Source: CAD feature listing. Evaluate the final solid. Frame: model axes, mm. A direction names the side the tool comes from. Round coordinates to 2 decimals unless told otherwise and drop trailing zeros. Order: outer loops, then holes, each group sorted by start corner. A loop starts at its lowest first (then second) coordinate and runs counter-clockwise, first axis right, second up. Notation, with made-up numbers: (27.5, 21) -> (35.5, 21) arc R28 cw to (35.5, 54) -> close; hole circle Ø4 at (-26.75, 1). An arc over 180 degrees is marked (long way). Write item = value, one per line. Start each with the question number.
(1) Cut plane C-C on y = 9.75. Return the cut outline in (x, z) (1 decimal).
(2) Draft query along X for faces 1 (the face through (31.8, -1.29, -38.16)), 2 (the face through (40, -1.787, -21)), 3 (the face through (28.797, 4.855, -34.608)). Return one class per face: released by +X, released by -X, zero draft, split by the parting line, or undercut.
(3) Cut plane A-A on y = 1.5. Give the number of separate pieces and of enclosed holes in the cut face, then the cut area to 3 significant figures.
(4) Cut plane B-B on x = 16. Return the cut outline in (y, z), then the cut area to 3 significant figures.
(5) Ray query, line 1 (X direction, y = 7, z = -19); line 2 (X direction, y = 1.5, z = -27.5); line 3 (Z direction, x = 21, y = 13.25). Return the intervals inside material, ascending.
(6) Contact query for flat-ended pins moving along their axis: pin 1 Ø6 at (y, z) = (10.5, -29.5) entering from -X; pin 2 Ø5.5 at (y, z) = (5.5, -22) entering from -X; pin 3 Ø1.4 at (x, z) = (4.5, -21.5) entering from +Y; pin 4 Ø4 at (x, z) = (8.5, -29) entering from +Y. Output: stop coordinate, or through.
(7) Reachability of faces 4 (the face through (30, 9.037, -6)), 5 (the face through (31.794, -1.294, -3.731)), 6 (the face through (14.534, 3.992, -13.953)) from +Z, -Z, +X, -X, +Y, -Y: full face, straight path, thin tool, end or side. Return the list, or none.
from build123d import *

# Parameters (mm, degrees)
BOSS_EXTRUDE1_DEPTH         = 0.7874
BOSS_EXTRUDE1_DEPTH_BACK    = 0.7874
SKETCH1_R                   = 20.955
SKETCH2_R                   = 1.8034
BOSS_EXTRUDE2_DEPTH         = 2.54
SKETCH3_R                   = 0.44958
BOSS_EXTRUDE3_DEPTH         = 12.7
CIRPATTERN1_COUNT           = 3
SKETCH4_R                   = 9.5
BOSS_EXTRUDE4_DEPTH         = 6.5
SKETCH5_W                   = 2.8
SKETCH5_H                   = 5
BOSS_EXTRUDE5_DEPTH         = 8.25
SKETCH6_R                   = 2
BOSS_EXTRUDE6_DEPTH         = 5.5
REVOLVE1_ANGLE              = 90
CIRPATTERN2_COUNT           = 6
SKETCH8_W                   = 1
SKETCH8_H                   = 3
BOSS_EXTRUDE7_DEPTH         = 1
SKETCH9_W                   = 2
SKETCH9_H                   = 2
BOSS_EXTRUDE8_DEPTH         = 1
FILLET1_R                   = 0.75
CIRPATTERN3_COUNT           = 6
FILLET1_OF_CIRPATTERN3_R    = 0.75
SKETCH11_W                  = 0.762
SKETCH11_H                  = 0.01
BOSS_EXTRUDE10_DEPTH        = 1.5748
CIRPATTERN4_COUNT           = 2
CIRPATTERN4_ANGLE           = 3.4725
CIRPATTERN5_COUNT           = 2
CIRPATTERN5_ANGLE           = 356.528
CIRPATTERN6_COUNT           = 3
CIRPATTERN6_COPY_1_SKETCH_W = 0.762
CIRPATTERN6_COPY_1_SKETCH_H = 0.01
CIRPATTERN6_COPY_1_DEPTH    = 1.5748
CIRPATTERN6_COPY_2_SKETCH_W = 0.762
CIRPATTERN6_COPY_2_SKETCH_H = 0.01
CIRPATTERN6_COPY_2_DEPTH    = 1.5748
CIRPATTERN6_COPY_3_SKETCH_W = 0.762
CIRPATTERN6_COPY_3_SKETCH_H = 0.01
CIRPATTERN6_COPY_3_DEPTH    = 1.5748
CIRPATTERN6_COPY_4_SKETCH_W = 0.762
CIRPATTERN6_COPY_4_SKETCH_H = 0.01
CIRPATTERN6_COPY_4_DEPTH    = 1.5748


with BuildPart() as part:
    # Sketch1 → Boss-Extrude1 (new, two sides: drawn at the far end of the back side and taken through both)
    with BuildSketch(Plane(origin=(0, 0, 0), x_dir=(1, 0, 0), z_dir=(0, 1, 0)).offset(-BOSS_EXTRUDE1_DEPTH_BACK)):
        with Locations(Location((20.955, 20.955, 0), (0, 0, 270))):
            Circle(SKETCH1_R)
    extrude(amount=BOSS_EXTRUDE1_DEPTH + BOSS_EXTRUDE1_DEPTH_BACK)

    # Sketch2 → Boss-Extrude2 (add)
    with BuildSketch(Plane(origin=(0, 0.7874, 0), x_dir=(1, 0, 0), z_dir=(0, 1, 0))):
        with Locations(Location((20.955, 5.842, 0), (0, 0, 270))):
            Circle(SKETCH2_R)
    boss_extrude2 = extrude(amount=BOSS_EXTRUDE2_DEPTH)

    # Sketch3 → Boss-Extrude3 (add)
    with BuildSketch(Plane(origin=(0, 3.3274, 0), x_dir=(1, 0, 0), z_dir=(0, 1, 0))):
        with Locations(Location((20.955, 5.842, 0), (0, 0, 270))):
            Circle(SKETCH3_R)
    boss_extrude3 = extrude(amount=BOSS_EXTRUDE3_DEPTH)

    # CirPattern1: Boss-Extrude2, Boss-Extrude3 ×3 about axis
    cirpattern1_axis = Axis((20.955, 0, -20.955), (0, 1, 0))
    add([boss_extrude2.rotate(cirpattern1_axis, i * 360 / CIRPATTERN1_COUNT) for i in range(1, CIRPATTERN1_COUNT)])
    add([boss_extrude3.rotate(cirpattern1_axis, i * 360 / CIRPATTERN1_COUNT) for i in range(1, CIRPATTERN1_COUNT)])

    # Sketch4 → Boss-Extrude4 (add)
    with BuildSketch(Plane(origin=(0, 0.7874, 0), x_dir=(1, 0, 0), z_dir=(0, 1, 0))):
        with Locations(Location((20.955, 20.955, 0), (0, 0, 90))):
            Circle(SKETCH4_R)
    extrude(amount=BOSS_EXTRUDE4_DEPTH)

    # Sketch5 → Boss-Extrude5 (add)
    with BuildSketch(Plane(origin=(0, 0.7874, 0), x_dir=(1, 0, 0), z_dir=(0, 1, 0))):
        with Locations((3.81, 20.955)):
            Rectangle(SKETCH5_W, SKETCH5_H)
    boss_extrude5 = extrude(amount=BOSS_EXTRUDE5_DEPTH)

    # Sketch6 → Boss-Extrude6 (add)
    with BuildSketch(Plane(origin=(0, 0.7874, 0), x_dir=(1, 0, 0), z_dir=(0, 1, 0))):
        with Locations((2.41, 20.955)):
            Circle(SKETCH6_R)
    boss_extrude6 = extrude(amount=BOSS_EXTRUDE6_DEPTH)

    # Sketch7 → Revolve1 (revolve)
    with BuildSketch(Plane(origin=(0, 6.2874, 0), x_dir=(1, 0, 0), z_dir=(0, 1, 0))):
        with BuildLine():
            Line((2.41, 22.955), (2.41, 18.955))
            ThreePointArc((2.41, 18.955), (0.41, 20.955), (2.41, 22.955))
        make_face()
    revolve1 = revolve(axis=Axis((2.41, 6.2874, -22.955), (0, 0, -1)), revolution_arc=REVOLVE1_ANGLE)

    # CirPattern2: Boss-Extrude5, Boss-Extrude6, Revolve1 ×6 about axis
    cirpattern2_axis = Axis((20.955, 0, -20.955), (0, 1, 0))
    add([boss_extrude5.rotate(cirpattern2_axis, i * 360 / CIRPATTERN2_COUNT) for i in range(1, CIRPATTERN2_COUNT)])
    add([boss_extrude6.rotate(cirpattern2_axis, i * 360 / CIRPATTERN2_COUNT) for i in range(1, CIRPATTERN2_COUNT)])
    add([revolve1.rotate(cirpattern2_axis, i * 360 / CIRPATTERN2_COUNT) for i in range(1, CIRPATTERN2_COUNT)])

    # Sketch8 → Boss-Extrude7 (add)
    with BuildSketch(Plane.XZ.offset(0.7874)):
        with Locations((1.905, -20.955)):
            Rectangle(SKETCH8_W, SKETCH8_H)
    boss_extrude7 = extrude(amount=BOSS_EXTRUDE7_DEPTH)

    # Sketch9 → Boss-Extrude8 (add)
    with BuildSketch(Plane.XZ.offset(0.7874)):
        with Locations((1.405, -20.955)):
            Rectangle(SKETCH9_W, SKETCH9_H)
    boss_extrude8 = extrude(amount=BOSS_EXTRUDE8_DEPTH)

    # Fillet1
    fillet1_edges = [part.edges().sort_by_distance(p)[0] for p in [
        (0.405, -1.2874, -21.955),
        (0.405, -1.2874, -19.955),
    ]]
    fillet(fillet1_edges, radius=FILLET1_R)

    # CirPattern3: Boss-Extrude7, Boss-Extrude8 ×6 about axis
    cirpattern3_axis = Axis((20.955, 0, -20.955), (0, 1, 0))
    add([boss_extrude7.rotate(cirpattern3_axis, i * 360 / CIRPATTERN3_COUNT) for i in range(1, CIRPATTERN3_COUNT)])
    add([boss_extrude8.rotate(cirpattern3_axis, i * 360 / CIRPATTERN3_COUNT) for i in range(1, CIRPATTERN3_COUNT)])

    # Fillet1 of CirPattern3
    fillet1_of_cirpattern3_edges = [part.edges().sort_by_distance(p)[0] for p in [
        (9.813974596, -1.2874, -3.658177952),
        (11.546025404, -1.2874, -2.658177952),
        (30.363974596, -1.2874, -2.658177952),
        (32.096025404, -1.2874, -3.658177952),
        (41.505, -1.2874, -19.955),
        (41.505, -1.2874, -21.955),
        (32.096025404, -1.2874, -38.251822048),
        (30.363974596, -1.2874, -39.251822048),
        (11.546025404, -1.2874, -39.251822048),
        (9.813974596, -1.2874, -38.251822048),
    ]]
    fillet(fillet1_of_cirpattern3_edges, radius=FILLET1_OF_CIRPATTERN3_R)

    # Sketch11 → Boss-Extrude10 (add)
    with BuildSketch(Plane(origin=(0, 0.7874, 0), x_dir=(-1, 0, 0), z_dir=(0, 1, 0))):
        with Locations((-20.955, -41.91)):
            Rectangle(SKETCH11_W, SKETCH11_H)
    boss_extrude10 = extrude(amount=-BOSS_EXTRUDE10_DEPTH)

    # CirPattern4: Boss-Extrude10 ×2 about axis
    cirpattern4_axis = Axis((20.955, 0, -20.955), (0, 1, 0))
    for i in range(1, CIRPATTERN4_COUNT):
        add(boss_extrude10.rotate(cirpattern4_axis, i * CIRPATTERN4_ANGLE / (CIRPATTERN4_COUNT - 1)))

    # CirPattern5: Boss-Extrude10 ×2 about axis
    cirpattern5_axis = Axis((20.955, 0.7874, -20.955), (0, 1, 0))
    for i in range(1, CIRPATTERN5_COUNT):
        add(boss_extrude10.rotate(cirpattern5_axis, i * CIRPATTERN5_ANGLE / (CIRPATTERN5_COUNT - 1)))

    # CirPattern6: Boss-Extrude10 ×3 about axis
    cirpattern6_axis = Axis((20.955, 0, -20.955), (0, 1, 0))
    for i in range(1, CIRPATTERN6_COUNT):
        add(boss_extrude10.rotate(cirpattern6_axis, i * 360 / CIRPATTERN6_COUNT))

    # CirPattern6 copy 1 sketch → CirPattern6 copy 1 (add)
    with BuildSketch(Plane(origin=(49.992077833, 0.7874, -15.032824647), x_dir=(0.5515366852909422, 0, 0.8341506367427168), z_dir=(0, 1, 0))):
        with Locations((-20.955, -41.91)):
            Rectangle(CIRPATTERN6_COPY_1_SKETCH_W, CIRPATTERN6_COPY_1_SKETCH_H)
    extrude(amount=-CIRPATTERN6_COPY_1_DEPTH)

    # CirPattern6 copy 2 sketch → CirPattern6 copy 2 (add)
    with BuildSketch(Plane(origin=(11.565215384, 0.7874, -49.062934732), x_dir=(0.4466272993566871, 0, -0.8947200989523774), z_dir=(0, 1, 0))):
        with Locations((-20.955, -41.91)):
            Rectangle(CIRPATTERN6_COPY_2_SKETCH_W, CIRPATTERN6_COPY_2_SKETCH_H)
    extrude(amount=-CIRPATTERN6_COPY_2_DEPTH)

    # CirPattern6 copy 3 sketch → CirPattern6 copy 3 (add)
    with BuildSketch(Plane(origin=(49.063016672, 0.7874, -11.565460673), x_dir=(0.44663510724549776, 0, 0.8947162013598516), z_dir=(0, 1, 0))):
        with Locations((-20.955, -41.91)):
            Rectangle(CIRPATTERN6_COPY_3_SKETCH_W, CIRPATTERN6_COPY_3_SKETCH_H)
    extrude(amount=-CIRPATTERN6_COPY_3_DEPTH)

    # CirPattern6 copy 4 sketch → CirPattern6 copy 4 (add)
    with BuildSketch(Plane(origin=(15.032571251, 0.7874, -49.992026151), x_dir=(0.551529405932396, 0, -0.834155449776514), z_dir=(0, 1, 0))):
        with Locations((-20.955, -41.91)):
            Rectangle(CIRPATTERN6_COPY_4_SKETCH_W, CIRPATTERN6_COPY_4_SKETCH_H)
    extrude(amount=-CIRPATTERN6_COPY_4_DEPTH)


solid = part.part
Evaluation:
q1.outline = circle Ø0.9 at (7.9, -28.5); circle Ø0.9 at (21, -5.8); circle Ø0.9 at (34, -28.5)
q2.face_1 = released by +X
q2.face_2 = zero draft
q2.face_3 = undercut
q3.separate_pieces = 10
q3.enclosed_holes = 0
q3.area = 436 mm^2
q4.outline = (-0.79, -41.32) -> (0.79, -41.32) -> (0.79, -29.06) -> (7.29, -29.06) -> (7.29, -12.85) -> (0.79, -12.85) -> (0.79, -0.59) -> (-0.79, -0.59) -> close
q4.area = 169 mm^2
q5.line_1 = 2.41 to 5.21, 11.66 to 30.25, 36.7 to 39.5
q5.line_2 = 6.37 to 9.36, 14.07 to 27.84, 32.55 to 35.54
q5.line_3 = -6.29 to -5.39
q6.pin_1 = 7.42
q6.pin_2 = 0.41
q6.pin_3 = 9.04
q6.pin_4 = 16.03
q7.face_4 = +Z, -Z, +X, +Y
q7.face_5 = +X, -Y
q7.face_6 = +Y
